from build123d import *

# Parameters (mm, degrees)
F1_W      = 5
F1_H      = 7.2
F1_H_2    = 6
F1_H_3    = 4
F1_W_2    = 23.3
F3_DEPTH  = 8.5
F4_DEPTH  = 23.2
F5_DEPTH  = 18.1
F6_START  = 4.3
F0_R      = 0.85
F6_DEPTH  = 20.7
F0_R_2    = 3.8
F7_DEPTH  = 5
F11_W     = 15
F11_H     = 11
F11_H_2   = 17
F11_W_2   = 4.6
F11_H_3   = 11.7
F11_W_3   = 28.7
F11_H_4   = 71.6
F12_DEPTH = 4
F13_DEPTH = 5
F14_DEPTH = 39
F16_R     = 3
F17_R     = 5
F15_R     = 1.985
F18_DEPTH = 10


with BuildPart() as f3:
    # F1 (on Front) → F3 (new body, symmetric)
    with BuildSketch(Plane.XZ):
        with Locations((-14.15, 13.6)):
            Rectangle(F1_W, F1_H)
        with Locations((-14.15, 20.2)):
            Rectangle(F1_W, F1_H_2)
        with Locations((-14.15, 7)):
            Rectangle(F1_W, F1_H_2)
        with Locations((-14.15, 2)):
            Rectangle(F1_W, F1_H_3)
        with Locations((0, 2)):
            Rectangle(F1_W_2, F1_H_3)
        with Locations((14.15, 2)):
            Rectangle(F1_W, F1_H_3)
        with Locations((14.15, 7)):
            Rectangle(F1_W, F1_H_2)
        with Locations((14.15, 13.6)):
            Rectangle(F1_W, F1_H)
        with Locations((14.15, 20.2)):
            Rectangle(F1_W, F1_H_2)
    extrude(amount=F3_DEPTH, both=True)

    # F0 (on Top) → F4 (join)
    with BuildSketch(Plane.XY):
        Polygon((11.65, 4.5), (11.65, 8.5), (0, 8.5), (-11.65, 8.5), (-11.65, 4.5), align=None)
    extrude(amount=F4_DEPTH)

    # F2 (on Right) → F5 (cut, symmetric)
    with BuildSketch(Plane.YZ):
        with BuildLine():
            Line((-8.5, 17.2), (-8.5, 10))
            Line((-8.5, 10), (3.5396314061, 10))
            ThreePointArc((3.5396314061, 10), (2.8089650426, 10.8020152096), (1.9224991399, 11.4275389379))
            Line((1.9224991399, 11.4275389379), (-5.9224991399, 15.7724610621))
            ThreePointArc((-5.9224991399, 15.7724610621), (-6.8089650426, 16.3979847904), (-7.5396314061, 17.2))
            Line((-7.5396314061, 17.2), (-8.5, 17.2))
        make_face()
        with BuildLine():
            Line((-8.5, 20.1464178425), (-8.5, 17.2))
            Line((-8.5, 17.2), (-7.5396314061, 17.2))
            ThreePointArc((-7.5396314061, 17.2), (-8.2538488107, 18.5969271247), (-8.5, 20.1464178425))
        make_face()
        with BuildLine():
            Line((-8.5, 10), (-8.5, 4))
            Line((-8.5, 4), (4.5, 4))
            Line((4.5, 4), (4.5, 7.0535821575))
            ThreePointArc((4.5, 7.0535821575), (4.2538488107, 8.6030728753), (3.5396314061, 10))
            Line((3.5396314061, 10), (-8.5, 10))
        make_face()
    extrude(amount=F5_DEPTH, both=True, mode=Mode.SUBTRACT)

    # F0 (on Top) → F6 (cut)
    with BuildSketch(Plane.XY.offset(F6_START)):
        with Locations((14.15, -2)):
            Circle(F0_R)
        with Locations((-14.15, -2)):
            Circle(F0_R)
    extrude(amount=F6_DEPTH, mode=Mode.SUBTRACT)

    # F0 (on Top) → F7 (join)
    with BuildSketch(Plane.XY):
        with Locations((5.75, -2.2)):
            Circle(F0_R_2)
    extrude(amount=-F7_DEPTH)


with BuildPart() as f3_1:
    # F8: moved
    add(f3.part.moved(Location((52.45, -56, 0))))


with BuildPart() as f9_1:
    # F9: instance of F3
    add(f3_1.part.mirror(Plane.XZ))


with BuildPart() as f10_1:
    # F10: instance of F9_1
    add(f9_1.part.mirror(Plane.YZ))


with BuildPart() as f10_2:
    # F10: instance of F3
    add(f3_1.part.mirror(Plane.YZ))


with BuildPart() as f3_2:
    add(f3_1.part)

    add(f9_1.part)  # F12 merges F9_1

    add(f10_1.part)  # F12 merges F10_1

    add(f10_2.part)  # F12 merges F10_2
    # F11 (on Top) → F12 (join)
    with BuildSketch(Plane.XY):
        Polygon((20.8, 47.5), (20.8, 64.5), (-20.8, 64.5), (-20.8, 47.5), (-20.8, 36.5), (-35.8, 36.5), (-35.8, 35.8), (-35.8, -35.8), (-35.8, -36.5), (-20.8, -36.5), (-20.8, -47.5), (-20.8, -64.5), (20.8, -64.5), (20.8, -47.5), (20.8, -36.5), (20.8, 36.5), align=None)
        with Locations((-28.3, -42)):
            Rectangle(F11_W, F11_H)
        with Locations((-28.3, -56)):
            Rectangle(F11_W, F11_H_2)
        Polygon((-35.8, -35.8), (-64.5, -35.8), (-64.5, -47.5), (-35.8, -47.5), (-35.8, -36.5), align=None)
        with Locations((-66.8, -41.65)):
            Rectangle(F11_W_2, F11_H_3)
        with Locations((-50.15, 0)):
            Rectangle(F11_W_3, F11_H_4)
        with Locations((-66.8, 0)):
            Rectangle(F11_W_2, F11_H_4)
        with Locations((28.3, -56)):
            Rectangle(F11_W, F11_H_2)
        with Locations((28.3, -42)):
            Rectangle(F11_W, F11_H)
        Polygon((64.5, -47.5), (64.5, -35.8), (35.8, -35.8), (35.8, -36.5), (35.8, -47.5), align=None)
        Polygon((64.5, -35.8), (64.5, 35.8), (35.8, 35.8), (35.8, 36.5), (20.8, 36.5), (20.8, -36.5), (35.8, -36.5), (35.8, -35.8), align=None)
        with Locations((66.8, 0)):
            Rectangle(F11_W_2, F11_H_4)
        with Locations((66.8, -41.65)):
            Rectangle(F11_W_2, F11_H_3)
        with Locations((28.3, 56)):
            Rectangle(F11_W, F11_H_2)
        with Locations((28.3, 42)):
            Rectangle(F11_W, F11_H)
        Polygon((64.5, 35.8), (64.5, 47.5), (35.8, 47.5), (35.8, 36.5), (35.8, 35.8), align=None)
        with Locations((66.8, 41.65)):
            Rectangle(F11_W_2, F11_H_3)
        with Locations((-28.3, 56)):
            Rectangle(F11_W, F11_H_2)
        with Locations((-28.3, 42)):
            Rectangle(F11_W, F11_H)
        Polygon((-35.8, 36.5), (-35.8, 47.5), (-64.5, 47.5), (-64.5, 35.8), (-35.8, 35.8), align=None)
        with Locations((-66.8, 41.65)):
            Rectangle(F11_W_2, F11_H_3)
    extrude(amount=F12_DEPTH)

    # F11 (on Top) → F13 (join)
    with BuildSketch(Plane.XY):
        Polygon((20.8, 47.5), (20.8, 64.5), (-20.8, 64.5), (-20.8, 47.5), (-20.8, 36.5), (-35.8, 36.5), (-35.8, 35.8), (-35.8, -35.8), (-35.8, -36.5), (-20.8, -36.5), (-20.8, -47.5), (-20.8, -64.5), (20.8, -64.5), (20.8, -47.5), (20.8, -36.5), (20.8, 36.5), align=None)
        with Locations((-50.15, 0)):
            Rectangle(F11_W_3, F11_H_4)
        with Locations((-66.8, 0)):
            Rectangle(F11_W_2, F11_H_4)
        with Locations((-28.3, -42)):
            Rectangle(F11_W, F11_H)
        with Locations((-28.3, -56)):
            Rectangle(F11_W, F11_H_2)
        with Locations((28.3, -56)):
            Rectangle(F11_W, F11_H_2)
        with Locations((28.3, -42)):
            Rectangle(F11_W, F11_H)
        Polygon((64.5, -35.8), (64.5, 35.8), (35.8, 35.8), (35.8, 36.5), (20.8, 36.5), (20.8, -36.5), (35.8, -36.5), (35.8, -35.8), align=None)
        with Locations((66.8, 0)):
            Rectangle(F11_W_2, F11_H_4)
        with Locations((28.3, 42)):
            Rectangle(F11_W, F11_H)
        with Locations((28.3, 56)):
            Rectangle(F11_W, F11_H_2)
        with Locations((-28.3, 56)):
            Rectangle(F11_W, F11_H_2)
        with Locations((-28.3, 42)):
            Rectangle(F11_W, F11_H)
    extrude(amount=-F13_DEPTH)

    # F11 (on Top) → F14 (join)
    with BuildSketch(Plane.XY):
        with Locations((-28.3, -56)):
            Rectangle(F11_W, F11_H_2)
        with Locations((-28.3, -42)):
            Rectangle(F11_W, F11_H)
        with Locations((28.3, -42)):
            Rectangle(F11_W, F11_H)
        with Locations((28.3, -56)):
            Rectangle(F11_W, F11_H_2)
        with Locations((28.3, 42)):
            Rectangle(F11_W, F11_H)
        with Locations((28.3, 56)):
            Rectangle(F11_W, F11_H_2)
        with Locations((-28.3, 42)):
            Rectangle(F11_W, F11_H)
        with Locations((-28.3, 56)):
            Rectangle(F11_W, F11_H_2)
    extrude(amount=F14_DEPTH)

    # F16
    f16_edges = [f3_2.edges().sort_by_distance(p)[0] for p in [
        (20.8, -50.5, 4),
        (20.8, 50.5, 4),
        (-20.8, 50.5, 4),
        (-20.8, -50.5, 4),
    ]]
    fillet(f16_edges, radius=F16_R)

    # F17
    f17_edges = [f3_2.edges().sort_by_distance(p)[0] for p in [
        (69.1, -64.5, 2),
        (69.1, 64.5, 2),
        (-69.1, 64.5, 2),
        (-69.1, -64.5, 2),
    ]]
    fillet(f17_edges, radius=F17_R)

    # F15 (on face) → F18 (cut)
    with BuildSketch(Plane.XY.offset(39)):
        with Locations((-28.3, -42)):
            Circle(F15_R)
        with Locations((28.3, -42)):
            Circle(F15_R)
        with Locations((28.3, 42)):
            Circle(F15_R)
        with Locations((-28.3, 42)):
            Circle(F15_R)
    extrude(amount=-F18_DEPTH, mode=Mode.SUBTRACT)


solid = f3_2.part
Geometry check sheet. Reference: the model listing, model coordinates, mm. A direction names the side the tool comes from. Round coordinates to 2 decimals unless told otherwise and drop trailing zeros. Order: outer loops, then holes, each group sorted by start corner. A loop starts at its lowest first (then second) coordinate and runs counter-clockwise, first axis right, second up. Notation, with made-up numbers: M 64,69 L 85,69 A15 cw 85,81 Z; hole C 32,28 d1. An arc over 180 degrees is marked long. Answer in a Markdown table with one row per item.
(1) Tool access check on faces 1 (the face through (19.94, 50.7, 4.9)), 2 (the face through (-52, 50, 23.2)), 3 (the face through (-64.1, 57, 19)). Record the directions out of +Z, -Z, +X, -X, +Y, -Y that give a thin tool (end or side, any length) a straight path to the whole face; none if there is none.
Responses:
| item | result |
|---|---|
| face 1 | +Z, +Y, -Y |
| face 2 | +Z, -X, +Y, -Y |
| face 3 | +Z, +Y |
(2) Sectioned sample at C-C, the plane y = -42. Record the cut outline in (x, z) (3 decimals).
Responses:
| item | result |
|---|---|
| outline | M -69.1,0 L -35.8,0 L -35.8,-5 L 35.8,-5 L 35.8,0 L 69.1,0 L 69.1,4 L 35.8,4 L 35.8,39 L 30.285,39 L 30.285,29 L 26.315,29 L 26.315,39 L 20.8,39 L 20.8,7 A3 cw 17.8,4 L -17.8,4 A3 cw -20.8,7 L -20.8,39 L -26.315,39 L -26.315,29 L -30.285,29 L -30.285,39 L -35.8,39 L -35.8,4 L -69.1,4 Z |
(3) Sectioned sample at D-D, the plane x = 14.5. Record the cut outline in (y, z).
Responses:
| item | result |
|---|---|
| outline | M -64.5,-5 L 64.5,-5 L 64.5,4 L -64.5,4 Z |
(4) Go/stop test with flat-tipped pins: P1, Ø4.5, axis at x = -28, y = 43, coming from the +Z side; P2, Ø1, axis at x = -38.3, y = 58, coming from the -Z side; P3, Ø2, axis at x = 27.5, y = -42.5, coming from the +Z side; P4, Ø15.5, axis at x = 57.5, z = 15, coming from the +Y side. Record where each tip stops, or that it passes through.
Responses:
| item | result |
|---|---|
| P1 | stops at z = 39 |
| P2 | stops at z = 0 |
| P3 | stops at z = 29 |
| P4 | stops at y = 64.38 |
(5) Sectioned sample at A-A, the plane z = 34. Record the cut outline in (x, y) (3 decimals), and give its area (3 significant figures).
Responses:
| item | result |
|---|---|
| outline | M -35.8,-64.5 L -20.8,-64.5 L -20.8,-36.5 L -35.8,-36.5 Z; M -35.8,36.5 L -20.8,36.5 L -20.8,64.5 L -35.8,64.5 Z; M 20.8,-64.5 L 35.8,-64.5 L 35.8,-36.5 L 20.8,-36.5 Z; M 20.8,36.5 L 35.8,36.5 L 35.8,64.5 L 20.8,64.5 Z; hole C -28.3,-42 d3.97; hole C -28.3,42 d3.97; hole C 28.3,-42 d3.97; hole C 28.3,42 d3.97 |
| area | 1,630 mm² |
(6) Draft check along Y on faces 4 (the face through (-54.404, -58.033, -2.465)), 5 (the face through (-27.23, -40.33, 34.07)), 6 (the face through (-53, 51.5, 13)), 7 (the face through (-35.8, 60, 8)). Enter one of: released by +Y, released by -Y, zero draft, split by the parting line, or undercut.
Responses:
| item | result |
|---|---|
| face 4 | undercut |
| face 5 | undercut |
| face 6 | released by +Y |
| face 7 | zero draft |
(7) Sectioned sample at B-B, the plane x = -58.2. Record the cut outline in (y, z), and give its area (3 significant figures).
Responses:
| item | result |
|---|---|
| outline | M -64.5,0 L -62,0 L -62,-5 L -54.4,-5 L -54.4,0 L -35.8,0 L -35.8,-5 L 35.8,-5 L 35.8,0 L 54.4,0 L 54.4,-5 L 62,-5 L 62,0 L 64.5,0 L 64.5,4 L 51.5,4 L 51.5,23.2 L 47.5,23.2 L 47.5,4 L -47.5,4 L -47.5,23.2 L -51.5,23.2 L -51.5,4 L -64.5,4 Z |
| area | 1,100 mm² |
(8) Scan lines: probe 1 along Y at (x, z) = (28.3, 35) (3 decimals); probe 2 along Y at (x, z) = (66.6, 18.25); probe 3 along Y at (x, z) = (-29.5, 20). Record each from-to range of solid material in increasing order. Write a range as from..to.
Responses:
| item | result |
|---|---|
| probe 1 | y = -64.5..-43.985, -40.015..-36.5, 36.5..40.015, 43.985..64.5 |
| probe 2 | y = -64.13..-58.85, -57.15..-47.5, 47.5..57.15, 58.85..64.13 |
| probe 3 | y = -64.5..-36.5, 36.5..64.5 |
